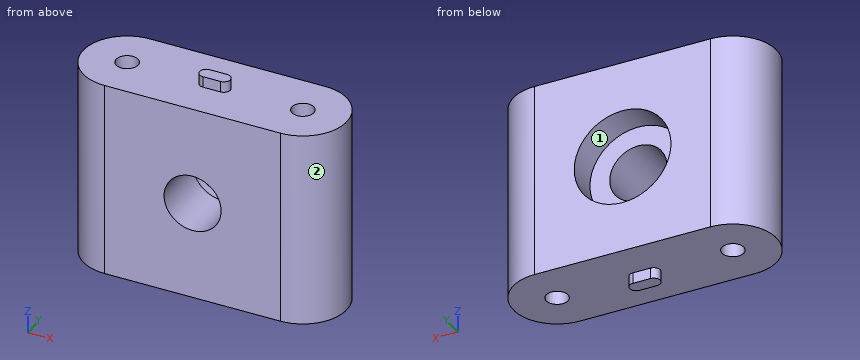
from build123d import *

# Parameters (mm, degrees)
SKETCH1_R                                   = 0.5
BOSS_EXTRUDE1_DEPTH                         = 4.5
BOSS_EXTRUDE2_DEPTH                         = 5
CBORE_FOR_M2_CHEESE_HEAD_SCREW1_D           = 2.6
CBORE_FOR_M2_CHEESE_HEAD_SCREW1_CBORE_D     = 4.4
CBORE_FOR_M2_CHEESE_HEAD_SCREW1_CBORE_DEPTH = 1.4


with BuildPart() as part:
    # Sketch1 → Boss-Extrude1 (new, symmetric)
    with BuildSketch(Plane.XY):
        with BuildLine():
            Line((-4, 2), (4, 2))
            ThreePointArc((4, 2), (6, 0), (4, -2))
            Line((4, -2), (-4, -2))
            ThreePointArc((-4, -2), (-6, 0), (-4, 2))
        make_face()
        with Locations((-4, 0)):
            Circle(SKETCH1_R, mode=Mode.SUBTRACT)
        with Locations((4, 0)):
            Circle(SKETCH1_R, mode=Mode.SUBTRACT)
        with BuildLine():
            Line((-0.4, 0.3), (0.4, 0.3))
            ThreePointArc((0.4, 0.3), (0.7, 0), (0.4, -0.3))
            Line((0.4, -0.3), (-0.4, -0.3))
            ThreePointArc((-0.4, -0.3), (-0.7, 0), (-0.4, 0.3))
        make_face(mode=Mode.SUBTRACT)
    extrude(amount=BOSS_EXTRUDE1_DEPTH, both=True)

    # Sketch1<2> → Boss-Extrude2 (add, symmetric)
    with BuildSketch(Plane.XY):
        with BuildLine():
            Line((-0.4, 0.3), (0.4, 0.3))
            ThreePointArc((0.4, 0.3), (0.7, 0), (0.4, -0.3))
            Line((0.4, -0.3), (-0.4, -0.3))
            ThreePointArc((-0.4, -0.3), (-0.7, 0), (-0.4, 0.3))
        make_face()
    extrude(amount=BOSS_EXTRUDE2_DEPTH, both=True)

    # CBORE for M2 Cheese Head Screw1 (through all)
    with Locations(Plane(origin=(0, 2, 0), x_dir=(1, 0, 0), z_dir=(0, 1, 0))):
        with Locations((0, 0)):
            CounterBoreHole(CBORE_FOR_M2_CHEESE_HEAD_SCREW1_D / 2, CBORE_FOR_M2_CHEESE_HEAD_SCREW1_CBORE_D / 2, CBORE_FOR_M2_CHEESE_HEAD_SCREW1_CBORE_DEPTH)


solid = part.part
Could you check a few things on this model? Use its own coordinates, in mm. Face numbers are marked on the shaded views. A direction names the side the tool comes from. Coordinates: 2 decimals unless noted, no trailing zeros. Loops run counter-clockwise (first coordinate to the right, second up) from the corner with the lowest first, then second, coordinate; pieces in that order, holes last. Notation, with made-up numbers: (72.5, -20) -> (77.5, -20) arc R16 ccw to (77.5, -1) -> close; hole circle Ø4 at (83.5, 68). An arc over 180 degrees is marked (long way). Answer in a Markdown table with one row per item.
(1) If I drill on probe 1 along X at (y, z) = (0.05, -4); probe 2 along Y at (x, z) = (4, -2.5); probe 3 along X at (y, z) = (0.2, 0.25), over which ranges is the centre line in solid material (lowest first)?
Results found:
| item | result |
|---|---|
| probe 1 | x = -6 to -4.5, -3.5 to 3.5, 4.5 to 6 |
| probe 2 | y = -2 to -0.5, 0.5 to 2 |
| probe 3 | x = -5.99 to -4.46, -3.54 to -1.28, 1.28 to 3.54, 4.46 to 5.99 |
(2) For the marked faces 1 and 2, which set-ups out of +Z, -Z, +X, -X, +Y, -Y let a thin tool reach every point of the face, with its end or its side?
Results found:
| item | result |
|---|---|
| face 1 | +Y |
| face 2 | +Z, -Z, +X |
(3) Imagine slicing it at B-B (z = 0). List the corners of the cut face in (x, y) for me.
Results found:
| item | result |
|---|---|
| outline | (-4, -2) -> (-1.3, -2) -> (-1.3, 0.6) -> (-2.2, 0.6) -> (-2.2, 2) -> (-4, 2) arc R2 ccw to start; (1.3, -2) -> (4, -2) arc R2 ccw to (4, 2) -> (2.2, 2) -> (2.2, 0.6) -> (1.3, 0.6) -> close; hole circle Ø1 at (-4, 0); hole circle Ø1 at (4, 0) |
(4) Imagine slicing it at C-C (x = 0). List the corners of the cut face in (y, z) for me.
Results found:
| item | result |
|---|---|
| outline | (-2, -4.5) -> (-0.3, -4.5) -> (-0.3, -5) -> (0.3, -5) -> (0.3, -4.5) -> (2, -4.5) -> (2, -2.2) -> (0.6, -2.2) -> (0.6, -1.3) -> (-2, -1.3) -> close; (-2, 1.3) -> (0.6, 1.3) -> (0.6, 2.2) -> (2, 2.2) -> (2, 4.5) -> (0.3, 4.5) -> (0.3, 5) -> (-0.3, 5) -> (-0.3, 4.5) -> (-2, 4.5) -> close |
(5) Imagine slicing it at D-D (z = 1.5). List the corners of the cut face in (x, y) for me, plus the area to 3 significant figures.
Results found:
| item | result |
|---|---|
| outline | (-4, -2) -> (4, -2) arc R2 ccw to (4, 2) -> (1.61, 2) -> (1.61, 0.6) -> (-1.61, 0.6) -> (-1.61, 2) -> (-4, 2) arc R2 ccw to start; hole circle Ø1 at (-4, 0); hole circle Ø1 at (4, 0) |
| area | 38.5 mm^2 |
(6) Will these pins go through, and if not, where does the flat tip stop? pin 1 Ø1.2 at (x, y) = (0.5, -1) entering from +Z; pin 2 Ø1.5 at (y, z) = (1, -2.5) entering from -X; pin 3 Ø1 at (x, y) = (-2.5, 0) entering from -Z.
Results found:
| item | result |
|---|---|
| pin 1 | stops at z = 4.5 |
| pin 2 | stops at x = -5.98 |
| pin 3 | stops at z = -4.5 |
(7) Imagine slicing it at A-A (y = 0). List the corners of the cut face in (x, z) for me, plus the area to 3 significant figures.
Results found:
| item | result |
|---|---|
| outline | (-6, -4.5) -> (-4.5, -4.5) -> (-4.5, 4.5) -> (-6, 4.5) -> close; (-3.5, -4.5) -> (-0.7, -4.5) -> (-0.7, -5) -> (0.7, -5) -> (0.7, -4.5) -> (3.5, -4.5) -> (3.5, 4.5) -> (0.7, 4.5) -> (0.7, 5) -> (-0.7, 5) -> (-0.7, 4.5) -> (-3.5, 4.5) -> close; (4.5, -4.5) -> (6, -4.5) -> (6, 4.5) -> (4.5, 4.5) -> close; hole circle Ø2.6 at (0, 0) |
| area | 86.1 mm^2 |
